For this review, take the finished solid that the model builds, in its own axes (mm). A direction names the side the tool comes from. Coordinates: 2 decimals unless noted, no trailing zeros. Loops run counter-clockwise (first coordinate to the right, second up) from the corner with the lowest first, then second, coordinate; pieces in that order, holes last.
```python
from build123d import *

# Parameters (mm, degrees)
F1_DEPTH = 12.7
F2_SIZE  = 5.08
F4_R     = 1.5875
F5_DEPTH = 11.73114
F6_SIZE  = 5.08
F8_DEPTH = 1.02158
F9_SIZE  = 0.254


with BuildPart() as f1:
    # F0 (on Front) → F1 (new body, symmetric)
    with BuildSketch(Plane.XZ):
        Polygon((-12.7, -38.581686), (0, -38.581686), (12.7, -38.581686), (12.7, -19.531686), (0, -19.531686), (-12.7, -19.531686), align=None)
    extrude(amount=F1_DEPTH, both=True)

    # F2
    f2_edges = [f1.edges().sort_by_distance(p)[0] for p in [
        (0, -12.7, -19.531686),
        (12.7, 0, -19.531686),
        (-12.7, 0, -19.531686),
        (0, 12.7, -19.531686),
        (-12.7, 0, -38.581686),
        (0, -12.7, -38.581686),
        (12.7, 0, -38.581686),
        (0, 12.7, -38.581686),
    ]]
    chamfer(f2_edges, length=F2_SIZE)

    # F4 (on offset) → F5 (join)
    with BuildSketch(Plane.XY.offset(-8.89)):
        Circle(F4_R)
    extrude(amount=-F5_DEPTH)

    # F6
    f6_edges = [f1.edges().sort_by_distance(p)[0] for p in [
        (-12.7, 12.7, -29.056686),
        (12.7, 12.7, -29.056686),
        (12.7, -12.7, -29.056686),
        (-12.7, -12.7, -29.056686),
    ]]
    chamfer(f6_edges, length=F6_SIZE)

    # F7 (on Right) → F8 (join, symmetric)
    with BuildSketch(Plane.YZ):
        Polygon((0.430685, -8.915657), (1.130668, -8.915657), (0, -6.847987), (-1.14363, -8.908516), (-0.443647, -8.908516), (0, -8.118563), align=None)
    extrude(amount=F8_DEPTH, both=True)

    # F9
    f9_edges = [f1.edges().sort_by_distance(p)[0] for p in [
        (0, 0, -6.847987),
    ]]
    chamfer(f9_edges, length=F9_SIZE)


solid = f1.part
```
Q1. For pin 1 Ø6 at (x, z) = (10, -29.5) entering from -Y; pin 2 Ø2 at (y, z) = (0, -8.5) entering from +X; pin 3 Ø0.5 at (y, z) = (0.5, -8) entering from -X; pin 4 Ø4 at (x, y) = (4, -2) entering from +Z, all flat-tipped, find the tip position at first contact; note any pin that passes through.
Q2. Machinability: for faces 4 (the face through (0, 12.7, -29)), 5 (the face through (-1.022, -0.024, -7.967)), 6 (the face through (-0.34, -1.55, -14.14)), 7 (the face through (1.022, -0.024, -7.967)), which of the approach directions +Z, -Z, +X, -X, +Y, -Y give a long, thin tool a straight path to every point of the face, cutting with its end or side? Answer none if there is none.
Q3. The part is to be moulded in two halves that separate along Y. For faces 1 (the face through (0, 0, -8.89)), 2 (the face through (2, 0, -19.532)), 3 (the face through (0.014, 0.626, -7.993)), say which applies: +Y half, -Y half, draft (parallel to the pull), parting line (faces both ways), or undercut.
Q4. Consider section C-C (y = -4.25). State the section outline as (x, z) points, then the cut area to 3 significant figures.
Q5. Consider section A-A (x = 0). State the section outline as (y, z) points.
Q6. Wall thickness on probe 1 along Z at (x, y) = (-3.5, -3); probe 2 along Z at (x, y) = (-6.75, 9.75); probe 3 along X at (y, z) = (-6, -36): over which ranges is each line inside the solid? List them lowest first.
Q7. Consider section B-B (z = -32). State the section outline as (x, y) points, then the cut area to 3 significant figures.
Q8. Consider section D-D (z = -15). State the section outline as (x, y) points (1 decimal).
Model answer:
1. pin 1: stops at y = -12.7
1. pin 2: stops at x = 1.59
1. pin 3: stops at x = -1.02
1. pin 4: stops at z = -19.53
2. face 4: +Z, -Z, +X, -X, +Y
2. face 5: +Z, -X, +Y, -Y
2. face 6: +Z
2. face 7: +Z, +X, +Y, -Y
3. face 1: undercut
3. face 2: draft
3. face 3: +Y half
4. outline: (-12.7, -33.5) - (-7.62, -38.58) - (7.62, -38.58) - (12.7, -33.5) - (12.7, -24.61) - (7.62, -19.53) - (-7.62, -19.53) - (-12.7, -24.61) - close
4. area: 432 mm2
5. outline: (-12.7, -33.5) - (-7.62, -38.58) - (7.62, -38.58) - (12.7, -33.5) - (12.7, -24.61) - (7.62, -19.53) - (1.59, -19.53) - (1.59, -8.89) - (1.12, -8.89) - (0.12, -7.07) - (-0.12, -7.07) - (-1.13, -8.89) - (-1.59, -8.89) - (-1.59, -19.53) - (-7.62, -19.53) - (-12.7, -24.61) - close; hole (-0.43, -8.89) - (0.42, -8.89) - (0, -8.12) - close
6. probe 1: z = -38.58 to -19.53
6. probe 2: z = -36.45 to -21.66
6. probe 3: x = -10.2 to 10.2
7. outline: (-12.7, -7.62) - (-7.62, -12.7) - (7.62, -12.7) - (12.7, -7.62) - (12.7, 7.62) - (7.62, 12.7) - (-7.62, 12.7) - (-12.7, 7.62) - close
7. area: 594 mm2
8. outline: circle Ø3.2 at (0, 0)
